Can you work these out from the model? Positions are in its coordinate system, mm. Face numbers are marked on the shaded views. A direction names the side the tool comes from. Give positions to 0.01 mm unless a question says otherwise; leave off trailing zeros. Loops run counter-clockwise (first coordinate to the right, second up) from the corner with the lowest first, then second, coordinate; pieces in that order, holes last. Notation, with made-up numbers: (77.5, -5.75) - (125.5, -5.75) arc R13 cw to (125.5, 1.25) - close; hole circle Ø11 at (12, -12). An arc over 180 degrees is marked (long way). Use a Markdown table: item, result. Add a question column.
```python
from build123d import *

# Parameters (mm, degrees)
SKETCH1_R               = 21
BOSS_EXTRUDE1_DEPTH     = 160
SKETCH3_W               = 65.933259094
SKETCH3_H               = 30
CUT_EXTRUDE3_DEPTH      = 17
CUT_EXTRUDE3_DEPTH_BACK = 57
CUT_EXTRUDE4_DEPTH      = 17
CUT_EXTRUDE4_DEPTH_BACK = 57
SKETCH6_W               = 300
SKETCH6_H               = 100
CUT_EXTRUDE5_DEPTH      = 17
CUT_EXTRUDE5_DEPTH_BACK = 57


with BuildPart() as part:
    # Sketch1 → Boss-Extrude1 (new body)
    with BuildSketch(Plane.XY):
        with BuildLine():
            Line((29.933259094, 20), (370.066740906, 20))
            ThreePointArc((370.066740906, 20), (436, 0), (370.066740906, -20))
            Line((370.066740906, -20), (29.933259094, -20))
            ThreePointArc((29.933259094, -20), (-36, 0), (29.933259094, 20))
        make_face()
        Circle(SKETCH1_R, mode=Mode.SUBTRACT)
        with Locations((400, 0)):
            Circle(SKETCH1_R, mode=Mode.SUBTRACT)
    extrude(amount=BOSS_EXTRUDE1_DEPTH)

    # Sketch3 → Cut-Extrude3 (cut, two sides)
    with BuildSketch(Plane(origin=(0, 20, 0), x_dir=(1, 0, 0), z_dir=(0, 1, 0))) as cut_extrude3_sk:
        Polygon((29.933259094, 0), (29.933259094, -30), (44.933259094, -30), (350, 0), align=None)
        with Locations((-3.033370453, -15)):
            Rectangle(SKETCH3_W, SKETCH3_H)
        with Locations((-3.033370453, -145)):
            Rectangle(SKETCH3_W, SKETCH3_H)
        Polygon((44.933259094, -130), (29.933259094, -130), (29.933259094, -160), (350, -160), align=None)
    extrude(amount=CUT_EXTRUDE3_DEPTH, mode=Mode.SUBTRACT)
    extrude(cut_extrude3_sk.sketch, amount=-CUT_EXTRUDE3_DEPTH_BACK, mode=Mode.SUBTRACT)

    # Sketch5 → Cut-Extrude4 (cut, two sides)
    with BuildSketch(Plane(origin=(0, 20, 0), x_dir=(1, 0, 0), z_dir=(0, 1, 0))) as cut_extrude4_sk:
        with BuildLine():
            Line((80, -63.737300936), (80, -96.262699064))
            ThreePointArc((80, -96.262699064), (85.181990285, -109.69499552), (98.042658808, -116.166689002))
            Line((98.042658808, -116.166689002), (222.553323511, -128.410960305))
            ThreePointArc((222.553323511, -128.410960305), (241.79037057, -122.053485026), (250, -103.530972882))
            Line((250, -103.530972882), (250, -56.469027118))
            ThreePointArc((250, -56.469027118), (241.79037057, -37.946514974), (222.553323511, -31.589039695))
            Line((222.553323511, -31.589039695), (98.042658808, -43.833310998))
            ThreePointArc((98.042658808, -43.833310998), (85.181990285, -50.30500448), (80, -63.737300936))
        make_face()
    extrude(amount=CUT_EXTRUDE4_DEPTH, mode=Mode.SUBTRACT)
    extrude(cut_extrude4_sk.sketch, amount=-CUT_EXTRUDE4_DEPTH_BACK, mode=Mode.SUBTRACT)

    # Sketch6 → Cut-Extrude5 (cut, two sides)
    with BuildSketch(Plane(origin=(0, 20, 0), x_dir=(1, 0, 0), z_dir=(0, 1, 0))) as cut_extrude5_sk:
        with Locations((436, -80)):
            Rectangle(SKETCH6_W, SKETCH6_H)
    extrude(amount=CUT_EXTRUDE5_DEPTH, mode=Mode.SUBTRACT)
    extrude(cut_extrude5_sk.sketch, amount=-CUT_EXTRUDE5_DEPTH_BACK, mode=Mode.SUBTRACT)


solid = part.part
```
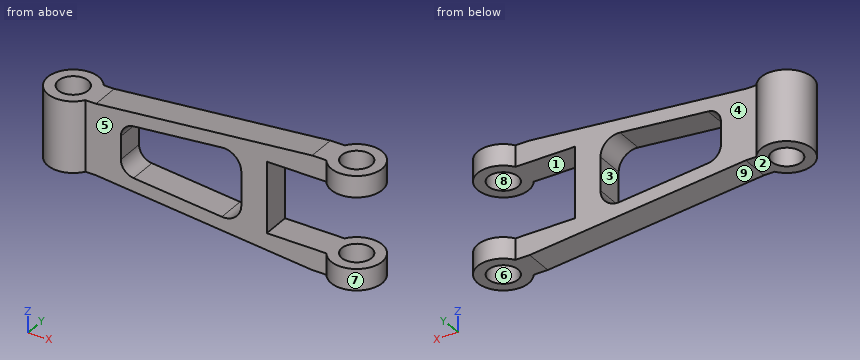
1. On a 3-axis mill with a long thin cutter (end or side, diameter ignored), from which of +Z, -Z, +X, -X, +Y, -Y can I reach the whole of each face in a straight line? I mean the marked faces 1, 2, 3, 4 and 5. Say none if no direction works.
2. Suppose I cut it at D-D (x = 400). List the corners of the cut face in (y, z) for me.
3. Suppose I cut it at A-A (z = 76). List the corners of the cut face in (x, y) for me.
4. Please list where these lines run through material, in increasing order: line 1 along Y through (x, z) = (400, 136); line 2 along X through (y, z) = (1, 57.5); line 3 along X through (y, z) = (0, 107). Write a range as [from, to].
5. If we mould it in two halves opening along Y, with no side actions, what happens to the marked faces 6, 7, 8 and 9? For each: released by +Y, released by -Y, zero draft, split by the parting line, or undercut.
6. Will these pins go through, and if not, where does the flat tip stop? P1, Ø2, axis at y = 3, z = 121, coming from the +X side; P2, Ø12, axis at x = 85, y = -22, coming from the +Z side; P3, Ø20, axis at y = 6, z = 73.5, coming from the -X side.
7. Suppose I cut it at C-C (x = 0). List the corners of the cut face in (y, z) for me, and give its area (3 significant figures).
8. Suppose I cut it at B-B (y = 0). State how many separate pieces and enclosed holes the cut face has, and give its area (3 significant figures).
Results below:
| question | item | result |
|---|---|---|
| 1 | face 1 | +X, +Y, -Y |
| 1 | face 2 | -Z, -X, +Y, -Y |
| 1 | face 3 | +Y, -Y |
| 1 | face 4 | +Z, -Z, +Y |
| 1 | face 5 | +Z, -Z, -Y |
| 2 | outline | (-36, 0) - (-21, 0) - (-21, 30) - (-36, 30) - close; (-36, 130) - (-21, 130) - (-21, 160) - (-36, 160) - close; (21, 0) - (36, 0) - (36, 30) - (21, 30) - close; (21, 130) - (36, 130) - (36, 160) - (21, 160) - close |
| 3 | outline | (29.93, -20) - (80, -20) - (80, 20) - (29.93, 20) arc R36 ccw (long way) to start; (250, -20) - (286, -20) - (286, 20) - (250, 20) - close; hole circle Ø42 at (0, 0) |
| 4 | line 1 | [-36, -21], [21, 36] |
| 4 | line 2 | [-35.99, -20.98], [20.98, 81], [250, 286] |
| 4 | line 3 | [-36, -21], [21, 83.13], [249.76, 286] |
| 5 | face 6 | undercut |
| 5 | face 7 | split by the parting line |
| 5 | face 8 | undercut |
| 5 | face 9 | zero draft |
| 6 | P1 | x = 286 |
| 6 | P2 | z = 134.5 |
| 6 | P3 | x = -36 |
| 7 | outline | (-36, 30) - (-21, 30) - (-21, 130) - (-36, 130) - close; (21, 30) - (36, 30) - (36, 130) - (21, 130) - close |
| 7 | area | 3,000 mm² |
| 8 | separate pieces | 4 |
| 8 | enclosed holes | 1 |
| 8 | area | 25,700 mm² |
